```python
from build123d import *

# Parameters (mm, degrees)
SKETCH1_W           = 67
SKETCH1_H           = 25.5
BOSS_EXTRUDE1_DEPTH = 2
SKETCH3_W           = 6
SKETCH3_H           = 25.5
BOSS_EXTRUDE2_DEPTH = 9
BOSS_EXTRUDE3_DEPTH = 9
SKETCH6_R           = 1.45
CUT_EXTRUDE1_DEPTH  = 3
CHAMFER1_SIZE       = 0.75
SKETCH7_R           = 1.05
CUT_EXTRUDE2_DEPTH  = 3


with BuildPart() as part:
    # Sketch1 → Boss-Extrude1 (new body)
    with BuildSketch(Plane(origin=(0, 0, 0), x_dir=(1, 0, 0), z_dir=(0, 1, 0))):
        with Locations((33.5, 12.75)):
            Rectangle(SKETCH1_W, SKETCH1_H)
    extrude(amount=BOSS_EXTRUDE1_DEPTH)

    # Sketch3 → Boss-Extrude2 (add)
    with BuildSketch(Plane(origin=(0, 2, 0), x_dir=(1, 0, 0), z_dir=(0, 1, 0))):
        with Locations((64, 12.75)):
            Rectangle(SKETCH3_W, SKETCH3_H)
    extrude(amount=BOSS_EXTRUDE2_DEPTH)

    # Sketch4 → Boss-Extrude3 (add)
    with BuildSketch(Plane(origin=(0, 2, 0), x_dir=(1, 0, 0), z_dir=(0, 1, 0))):
        Polygon((0, 0), (6, 0), (6, 12.5), (4.5, 12.5), (4.5, 16.75), (6, 16.75), (6, 25.5), (0, 25.5), align=None)
    extrude(amount=BOSS_EXTRUDE3_DEPTH)

    # Sketch6 → Cut-Extrude1 (cut)
    with BuildSketch(Plane(origin=(0, 11, 0), x_dir=(1, 0, 0), z_dir=(0, 1, 0))):
        with Locations(Location((2.911463201, 22.5, 0), (0, 0, 270))):
            Circle(SKETCH6_R)
        with Locations(Location((2.988195093, 3, 0), (0, 0, 270))):
            Circle(SKETCH6_R)
        with Locations(Location((64, 22.5, 0), (0, 0, 270))):
            Circle(SKETCH6_R)
        with Locations(Location((64, 3, 0), (0, 0, 270))):
            Circle(SKETCH6_R)
    extrude(amount=-CUT_EXTRUDE1_DEPTH, mode=Mode.SUBTRACT)

    # Chamfer1
    chamfer1_edges = [part.edges().sort_by_distance(p)[0] for p in [
        (61, 2, -12.75),
        (67, 11, -12.75),
        (61, 11, -12.75),
        (6, 2, -6.25),
        (6, 2, -21.125),
        (0, 11, -12.75),
        (6, 11, -6.25),
        (6, 11, -21.125),
        (67, 0, -12.75),
        (0, 0, -12.75),
    ]]
    chamfer(chamfer1_edges, length=CHAMFER1_SIZE)

    # Sketch7 → Cut-Extrude2 (cut)
    with BuildSketch(Plane(origin=(0, 8, 0), x_dir=(1, 0, 0), z_dir=(0, 1, 0))):
        with Locations(Location((2.911463201, 22.5, 0), (0, 0, 270))):
            Circle(SKETCH7_R)
        with Locations(Location((2.988195093, 3, 0), (0, 0, 270))):
            Circle(SKETCH7_R)
        with Locations(Location((64, 3, 0), (0, 0, 270))):
            Circle(SKETCH7_R)
        with Locations(Location((64, 22.5, 0), (0, 0, 270))):
            Circle(SKETCH7_R)
    extrude(amount=-CUT_EXTRUDE2_DEPTH, mode=Mode.SUBTRACT)


solid = part.part
```
Work out the finished part from the listing and answer in its coordinate system (mm). A direction names the side the tool comes from. Coordinates: 2 decimals unless noted, no trailing zeros. Loops run counter-clockwise (first coordinate to the right, second up) from the corner with the lowest first, then second, coordinate; pieces in that order, holes last. Notation, with made-up numbers: M -10.75,81.25 L 24.25,81.25 A25 cw 24.25,107.25 Z; hole C 75.25,76 d4. An arc over 180 degrees is marked long. Use CSV: the item, a comma, the result in double quotes. Start each with the question number.
(1) Find section C-C, the plane x = 64. Give the vertices of the cut face in (y, z).
(2) Given pin 1 Ø6 at (x, z) = (41.5, -4.5) entering from +Y; pin 2 Ø1.7 at (x, z) = (64, -22.5) entering from +Y; pin 3 Ø6 at (x, y) = (41, 6) entering from -Z, each flat-ended and moving along its own axis, determine where each tip first touches the part or whether it passes through.
(3) For a pull along X with two mould halves and no side action, classify faces 1 (the face through (33, 0, -13)), 2 (the face through (67, 5, -13)), 3 (the face through (3.968, 9.521, -4.069)) as +X half, -X half, draft (parallel to the pull), parting line (faces both ways), or undercut.
(4) Find section B-B, the plane y = 8.75. Give the vertices of the cut face in (x, z), then the cut area to 3 significant figures.
(5) Find section A-A, the plane z = -11.75. Give the vertices of the cut face in (x, y), then the cut area to 3 significant figures.
(6) Consider line 1 (X direction, y = 5.7, z = -22.5); line 2 (X direction, y = 8.85, z = -3); line 3 (Z direction, x = 64, y = 8.5). Determine where each line is inside the solid, lowest interval first.
(7) For faces 4 (the face through (6, 6, -21)), 5 (the face through (4.5, 6, -15)), 6 (the face through (3, 11, -13)), determine the directions among +Z, -Z, +X, -X, +Y, -Y from which every point of the face is accessible in a straight line to the end or side of a thin tool.
Recorded:
1,outline,"M 0,-25.5 L 11,-25.5 L 11,-23.95 L 8,-23.95 L 8,-23.55 L 5,-23.55 L 5,-21.45 L 8,-21.45 L 8,-21.05 L 11,-21.05 L 11,-4.45 L 8,-4.45 L 8,-4.05 L 5,-4.05 L 5,-1.95 L 8,-1.95 L 8,-1.55 L 11,-1.55 L 11,0 L 0,0 Z"
2,pin 1,"stops at y = 2"
2,pin 2,"stops at y = 5"
2,pin 3,"passes through"
3,face 1,"draft"
3,face 2,"+X half"
3,face 3,"undercut"
4,outline,"M 0,-25.5 L 6,-25.5 L 6,-16.75 L 4.5,-16.75 L 4.5,-12.5 L 6,-12.5 L 6,0 L 0,0 Z; M 61,-25.5 L 67,-25.5 L 67,0 L 61,0 Z; hole C 2.91,-22.5 d2.9; hole C 2.99,-3 d2.9; hole C 64,-22.5 d2.9; hole C 64,-3 d2.9"
4,area,"273 mm^2"
5,outline,"M 0,0.75 L 0.75,0 L 66.25,0 L 67,0.75 L 67,10.25 L 66.25,11 L 61.75,11 L 61,10.25 L 61,2.75 L 60.25,2 L 6.75,2 L 6,2.75 L 6,10.25 L 5.25,11 L 0.75,11 L 0,10.25 Z"
5,area,"241 mm^2"
6,line 1,"x = 0 to 1.86, 3.96 to 6, 61 to 62.95, 65.05 to 67"
6,line 2,"x = 0 to 1.54, 4.44 to 6, 61 to 62.55, 65.45 to 67"
6,line 3,"z = -25.5 to -23.95, -21.05 to -4.45, -1.55 to 0"
7,face 4,"+Z, -Z, +Y"
7,face 5,"+Y"
7,face 6,"+Z, -Z, +X, -X, +Y"
